Model file for the job. Use its own axes, mm. Give positions to 0.01 mm unless a question says otherwise; leave off trailing zeros. Order: outer loops, then holes, each group sorted by start corner. A loop starts at its lowest first (then second) coordinate and runs counter-clockwise, first axis right, second up. Notation, with made-up numbers: M 21,26 L 25,26 A12 cw 25,36 Z; hole C 57,29 d9. An arc over 180 degrees is marked long. Return JSON: item names as keys, results as strings. Group by question number.
1. Slice it at A-A on x = 87. List the corners of the cut face in (y, z), then the cut area to 3 significant figures.
2. Pin check, flat tips, straight feed: pin 1 (1 mm diameter, centred on y = 128, z = 125.5, fed in from -X); pin 2 (1 mm diameter, centred on y = 149.5, z = 126, fed in from +X); pin 3 (1 mm diameter, centred on x = 89.5, y = 135, fed in from -Z). Stop position of each tip, or through.
3. Slice it at C-C on y = 177.5. List the corners of the cut face in (x, z), then the cut area to 3 significant figures.
4. Wall check: probe 1 along Z at (x, y) = (88, 159); probe 2 along Y at (x, z) = (88, 123.5); probe 3 along X at (y, z) = (200, 128). Give the ranges that are in metal, low to high. Write a range as [from, to].
5. Two-plate mould, pull along X, no slides. Class faces 1 (the face through (85, 96.451, 124)), 2 (the face through (82.735, 152.221, 127.588)), 3 (the face through (86, 109, 132)): released by +X, released by -X, zero draft, split by the parting line, or undercut.
6. Slice it at B-B on z = 128.75. List the corners of the cut face in (x, y), then the cut area to 3 significant figures.
from build123d import *

# Parameters (mm, degrees)
SKETCH1_R                = 5
SKETCH1_R_2              = 4
BOSS_EXTRUDE1_DEPTH      = 80
BOSS_EXTRUDE1_DEPTH_BACK = 30
SKETCH2_R                = 3
CUT_EXTRUDE1_DEPTH       = 6
CUT_EXTRUDE1_DEPTH_BACK  = 6


with BuildPart() as part:
    # Sketch1 → Boss-Extrude1 (new body, two sides)
    with BuildSketch(Plane(origin=(0, 126.450796526, 0), x_dir=(1, 0, 0), z_dir=(0, 1, 0))) as boss_extrude1_sk:
        with Locations((87.72987116, -127.807872395)):
            Circle(SKETCH1_R)
        with Locations((87.72987116, -127.807872395)):
            Circle(SKETCH1_R_2, mode=Mode.SUBTRACT)
    extrude(amount=BOSS_EXTRUDE1_DEPTH)
    extrude(boss_extrude1_sk.sketch, amount=-BOSS_EXTRUDE1_DEPTH_BACK)

    # Sketch2 → Cut-Extrude1 (cut, two sides)
    with BuildSketch(Plane(origin=(-5.567034038, 0.110667347, 127.807872395), x_dir=(-1, 0, 0), z_dir=(0, 0, -1))) as cut_extrude1_sk:
        with Locations((-93.296905198, 111.340129179)):
            Circle(SKETCH2_R)
    extrude(amount=CUT_EXTRUDE1_DEPTH, mode=Mode.SUBTRACT)
    extrude(cut_extrude1_sk.sketch, amount=-CUT_EXTRUDE1_DEPTH_BACK, mode=Mode.SUBTRACT)


solid = part.part
Result:
{
 "1": {"outline": "M 96.45,122.86 L 108.54,122.86 L 108.54,123.88 L 96.45,123.88 Z; M 96.45,131.74 L 108.54,131.74 L 108.54,132.75 L 96.45,132.75 Z; M 114.36,122.86 L 206.45,122.86 L 206.45,123.88 L 114.36,123.88 Z; M 114.36,131.74 L 206.45,131.74 L 206.45,132.75 L 114.36,132.75 Z", "area": "211 mm2"},
 "2": {"pin 1": "stops at x = 83.07", "pin 2": "stops at x = 92.56", "pin 3": "stops at z = 122.97"},
 "3": {"outline": "C 87.73,127.81 d10; hole C 87.73,127.81 d8", "area": "28.3 mm2"},
 "4": {"probe 1": "z = [122.82, 123.82], [131.8, 132.8]", "probe 2": "y = [96.45, 108.46], [114.44, 206.45]", "probe 3": "x = [82.73, 83.73], [91.73, 92.73]"},
 "5": {"face 1": "zero draft", "face 2": "split by the parting line", "face 3": "undercut"},
 "6": {"outline": "M 82.82,96.45 L 83.84,96.45 L 83.84,206.45 L 82.82,206.45 Z; M 91.62,96.45 L 92.64,96.45 L 92.64,206.45 L 91.62,206.45 Z", "area": "225 mm2"}
}
